```python
from build123d import *

# Parameters (mm, degrees)
BOSS_EXTRUDE1_DEPTH = 1700
SCALE1_SCALE        = 0.75


with BuildPart() as part:
    # Sketch1 → Boss-Extrude1 (new body)
    with BuildSketch(Plane.XY.offset(1800)):
        with BuildLine():
            Line((129, 60.46884946), (129, 30))
            Line((129, 30), (124.919748757, 30))
            Line((124.919748757, 30), (122.792728308, 12.689402566))
            ThreePointArc((122.792728308, 12.689402566), (119.171200489, 5.771495525), (111.871083085, 3))
            Line((111.871083085, 3), (-1.871083085, 3))
            ThreePointArc((-1.871083085, 3), (-9.171200492, 5.771495528), (-12.792728309, 12.689402573))
            Line((-12.792728309, 12.689402573), (-18.294338419, 58.536153493))
            ThreePointArc((-18.294338419, 58.536153493), (-19.775872526, 61.366206375), (-22.762284192, 62.5))
            Line((-22.762284192, 62.5), (-25, 62.5))
            Line((-25, 62.5), (-25, -62.5))
            Line((-25, -62.5), (-22.762284192, -62.5))
            ThreePointArc((-22.762284192, -62.5), (-19.775872526, -61.366206375), (-18.294338419, -58.536153493))
            Line((-18.294338419, -58.536153493), (-12.792728309, -12.689402573))
            ThreePointArc((-12.792728309, -12.689402573), (-9.171200492, -5.771495528), (-1.871083085, -3))
            Line((-1.871083085, -3), (111.871083085, -3))
            ThreePointArc((111.871083085, -3), (119.171200492, -5.771495528), (122.792728309, -12.689402573))
            Line((122.792728309, -12.689402573), (124.87, -30))
            Line((124.87, -30), (129, -30))
            Line((129, -30), (129, -60.46884946))
            ThreePointArc((129, -60.46884946), (130.62450761, -61.959786773), (132.762284192, -62.5))
            Line((132.762284192, -62.5), (135, -62.5))
            Line((135, -62.5), (135, 62.5))
            Line((135, 62.5), (132.762284192, 62.5))
            ThreePointArc((132.762284192, 62.5), (130.62450761, 61.959786773), (129, 60.46884946))
        make_face()
    extrude(amount=-BOSS_EXTRUDE1_DEPTH)


with BuildPart() as part_1:
    # Scale1: scaled about (51.838667986, -0.00324275, 950)
    add(part.part.scale(SCALE1_SCALE).moved(Location((12.959666996, -0.000810687, 237.5))))


solid = part_1.part
```
Part model, mm, in its own coordinate system. A direction names the side the tool comes from. Coordinates: 2 decimals unless noted, no trailing zeros. Order: outer loops, then holes, each group sorted by start corner. A loop starts at its lowest first (then second) coordinate and runs counter-clockwise, first axis right, second up. Notation, with made-up numbers: (52.5, -12.5) -> (73.5, -12.5) arc R17 ccw to (73.5, -0.5) -> close; hole circle Ø9 at (19, 23). An arc over 180 degrees is marked (long way). Put each result on its own line as item: value. Start each with the question number.
(1) Band-saw the part on B-B (x = 75). Give the cut face in (y, z).
(2) Band-saw the part on A-A (z = 1314). Give the cut face in (x, y) (3 decimals), then the cut area to 3 significant figures.
(3) Mould opens along X. For faces 4 (the face through (-5.79, 1, 959)), 5 (the face through (1.33, 26.47, 958.92)), 6 (the face through (54, 0, 1587.5)) say: pulls with the +X half, pulls with the -X half, needs draft (parallel to the pull), parting line crosses it, or undercut.
(4) Pin check, flat tips, straight feed: pin 1 Ø5 at (x, z) = (63.5, 1198.5) entering from +Y; pin 2 Ø5 at (x, z) = (99, 511) entering from -Y; pin 3 Ø6 at (x, z) = (64.5, 1395.5) entering from -Y. Stop position of each tip, or through.
(5) Which spindle directions (+Z, -Z, +X, -X, +Y, -Y) get a long thin tool onto all of the face, cutting with end or side? Do faces 1 (the face through (109.71, 34, 959)), 2 (the face through (1.273, -26.951, 958.925)), 3 (the face through (54, 0, 312.5)). Say none if no direction does.
(6) Probe line 1 along Y through (x, z) = (10.5, 609); line 2 along X through (y, z) = (-27.5, 859.5); line 3 along Y through (x, z) = (19.5, 1249). List the from-to ranges inside material, lowest first. Write a range as [from, to].
Determined:
1. outline: (-2.25, 312.5) -> (2.25, 312.5) -> (2.25, 1587.5) -> (-2.25, 1587.5) -> close
2. outline: (-5.79, -46.876) -> (-4.112, -46.876) arc R3.375 ccw to (-0.761, -43.903) -> (3.365, -9.518) arc R8.25 cw to (11.556, -2.251) -> (96.863, -2.251) arc R8.25 cw to (105.054, -9.518) -> (106.612, -22.501) -> (109.71, -22.501) -> (109.71, -45.352) arc R3.375 ccw to (112.531, -46.876) -> (114.21, -46.876) -> (114.21, 46.874) -> (112.531, 46.874) arc R3.375 ccw to (109.71, 45.351) -> (109.71, 22.499) -> (106.649, 22.499) -> (105.054, 9.516) arc R8.25 cw to (96.863, 2.249) -> (11.556, 2.249) arc R8.25 cw to (3.365, 9.516) -> (-0.761, 43.901) arc R3.375 ccw to (-4.112, 46.874) -> (-5.79, 46.874) -> close
2. area: 1,810 mm²
3. face 4: pulls with the -X half
3. face 5: undercut
3. face 6: needs draft
4. pin 1: stops at y = 2.25
4. pin 2: stops at y = -3.68
4. pin 3: stops at y = -2.25
5. face 1: +Z, -Z, +Y
5. face 2: +Z, -Z, -Y
5. face 3: -Z, +X, -X, +Y, -Y
6. line 1: y = [-2.32, 2.32]
6. line 2: x = [-5.79, 1.21], [109.71, 114.21]
6. line 3: y = [-2.25, 2.25]
